Geometry check sheet. Reference: the model listing, model coordinates, mm. Face numbers are marked on the shaded views. Give positions to 0.01 mm unless a question says otherwise; leave off trailing zeros. Write each loop counter-clockwise with the first axis right and the second up, starting at its lowest first coordinate (ties: lowest second). Pieces come first, ordered by that corner, then holes. Notation, with made-up numbers: (65.5, 87) - (106.5, 87) arc R17 cw to (106.5, 118) - close; hole circle Ø10 at (-34.75, -28.75). An arc over 180 degrees is marked (long way). Use a Markdown table: item, result.
```python
from build123d import *

# Parameters (mm, degrees)
BOSS_EXTRUDE1_DEPTH = 5.08
CAVITY2_OUTLINE_R   = 4.59774385
CAVITY2_OUTLINE_R_2 = 13.7414
CAVITY2_DEPTH       = 4.3688
CAVITY2_START       = 3.2512
CAVITY2_2_DEPTH     = 1.1176
CAVITY2_3_OUTLINE_R = 2.794
CAVITY2_3_DEPTH     = 0.7112
SKETCH10_R          = 4.59774385
SKETCH10_R_2        = 2.794
CUT_EXTRUDE1_DEPTH  = 5.08


# Read off the part's stored shape, not the designer's step: Cavity2
with BuildPart() as part:
    # Sketch1 → Boss-Extrude1 (new body)
    with BuildSketch(Plane.XY):
        Polygon((-94.341860078, 47.544254219), (-72.328526744, 47.544254219), (-72.328526744, 52.624254219), (-53.278526744, 52.624254219), (-53.278526744, 47.544254219), (-31.265193411, 47.544254219), (-31.265193411, 52.624254219), (-12.215193411, 52.624254219), (-12.215193411, 47.544254219), (9.798139922, 47.544254219), (9.798139922, 26.589254219), (14.878139922, 26.589254219), (14.878139922, 7.539254219), (9.798139922, 7.539254219), (9.798139922, -13.415745781), (-94.341860078, -13.415745781), (-94.341860078, 7.539254219), (-99.421860078, 7.539254219), (-99.421860078, 26.589254219), (-94.341860078, 26.589254219), align=None)
    extrude(amount=BOSS_EXTRUDE1_DEPTH)

    # Cavity2 outline → Cavity2 (cut)
    with BuildSketch(Plane.XY):
        with Locations((-53.811820296, 33.77125273)):
            Circle(CAVITY2_OUTLINE_R)
        with Locations((-72.649126193, 23.706396)):
            Circle(CAVITY2_OUTLINE_R_2)
    extrude(amount=CAVITY2_DEPTH, mode=Mode.SUBTRACT)

    # Cavity2 2 outline → Cavity2 2 (cut)
    with BuildSketch(Plane.XY.offset(CAVITY2_START)):
        with BuildLine():
            Line((-85.401408895, 28.825513097), (-90.989734661, 27.7567927))
            Line((-90.989734661, 27.7567927), (-88.279765083, 13.586395221))
            Line((-88.279765083, 13.586395221), (-82.945631867, 14.606503426))
            ThreePointArc((-82.945631867, 14.606503426), (-86.190053798, 21.367731092), (-85.401408895, 28.825513097))
        make_face()
    extrude(amount=CAVITY2_2_DEPTH, mode=Mode.SUBTRACT)

    # Cavity2 3 outline → Cavity2 3 (cut)
    with BuildSketch(Plane.XY):
        with Locations((-27.031860078, 2.217954219)):
            Circle(CAVITY2_3_OUTLINE_R)
    extrude(amount=CAVITY2_3_DEPTH, mode=Mode.SUBTRACT)

    # Sketch10 → Cut-Extrude1 (cut)
    with BuildSketch(Plane(origin=(0, 0, 0), x_dir=(-1, 0, 0), z_dir=(0, 0, -1))):
        with Locations((53.811820296, 33.77125273)):
            Circle(SKETCH10_R)
        with Locations((27.031860078, 2.217954219)):
            Circle(SKETCH10_R_2)
        with BuildLine():
            Line((82.945631867, 14.606503426), (88.279765083, 13.586395221))
            Line((88.279765083, 13.586395221), (90.989734661, 27.7567927))
            Line((90.989734661, 27.7567927), (85.401408894, 28.825513097))
            ThreePointArc((85.401408894, 28.825513097), (59.108198587, 26.045060907), (82.945631867, 14.606503426))
        make_face()
    extrude(amount=-CUT_EXTRUDE1_DEPTH, mode=Mode.SUBTRACT)


solid = part.part
```
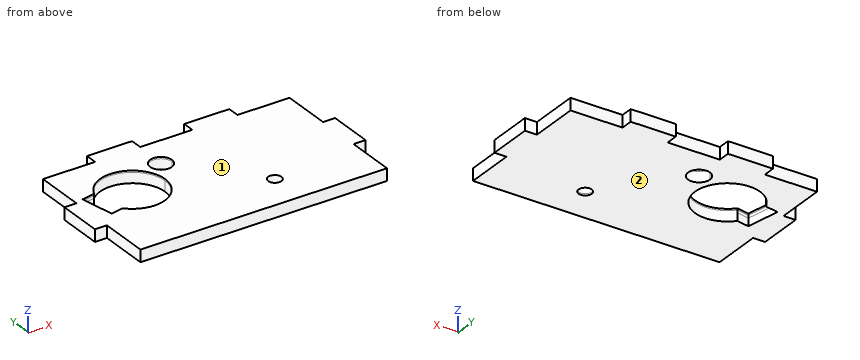
1) Section check D-D on y = 36. Record the boundary of the cut face in (x, z), then the cut area to 3 significant figures.
Working result:
| item | result |
|---|---|
| outline | (-94.34, 0) - (-78.79, 0) - (-78.79, 5.08) - (-94.34, 5.08) - close; (-66.51, 0) - (-57.83, 0) - (-57.83, 5.08) - (-66.51, 5.08) - close; (-49.79, 0) - (9.8, 0) - (9.8, 5.08) - (-49.79, 5.08) - close |
| area | 426 mm² |
2) Mould release check, pull along Z, two halves, no side actions. Record for the marked faces 1 and 2: pulls with the +Z half, pulls with the -Z half, needs draft (parallel to the pull), parting line crosses it, or undercut.
Working result:
| item | result |
|---|---|
| face 1 | pulls with the +Z half |
| face 2 | pulls with the -Z half |
3) Material ranges on L1, parallel to X at y = 49.5, z = 3.65; L2, parallel to X at y = 2, z = 1.35; L3, parallel to X at y = 30, z = 2.1, recorded low to high. Write a range as from..to.
Working result:
| item | result |
|---|---|
| L1 | x = -72.33..-53.28, -31.27..-12.22 |
| L2 | x = -94.34..-29.82, -24.25..9.8 |
| L3 | x = -94.34..-84.86, -60.43..-56.44, -51.18..9.8 |
4) Section check A-A on y = 49. Record the boundary of the cut face in (x, z), then the cut area to 3 significant figures.
Working result:
| item | result |
|---|---|
| outline | (-72.33, 0) - (-53.28, 0) - (-53.28, 5.08) - (-72.33, 5.08) - close; (-31.27, 0) - (-12.22, 0) - (-12.22, 5.08) - (-31.27, 5.08) - close |
| area | 194 mm² |
5) Section check B-B on x = -63. Record the boundary of the cut face in (y, z), then the cut area to 3 significant figures.
Working result:
| item | result |
|---|---|
| outline | (-13.42, 0) - (13.92, 0) - (13.92, 5.08) - (-13.42, 5.08) - close; (33.49, 0) - (52.62, 0) - (52.62, 5.08) - (33.49, 5.08) - close |
| area | 236 mm² |
6) Section check C-C on z = 1.55. Record the boundary of the cut face in (x, y).
Working result:
| item | result |
|---|---|
| outline | (-99.42, 7.54) - (-94.34, 7.54) - (-94.34, -13.42) - (9.8, -13.42) - (9.8, 7.54) - (14.88, 7.54) - (14.88, 26.59) - (9.8, 26.59) - (9.8, 47.54) - (-12.22, 47.54) - (-12.22, 52.62) - (-31.27, 52.62) - (-31.27, 47.54) - (-53.28, 47.54) - (-53.28, 52.62) - (-72.33, 52.62) - (-72.33, 47.54) - (-94.34, 47.54) - (-94.34, 26.59) - (-99.42, 26.59) - close; hole (-90.99, 27.76) - (-88.28, 13.59) - (-82.95, 14.61) arc R13.74 ccw (long way) to (-85.4, 28.83) - close; hole circle Ø9.2 at (-53.81, 33.77); hole circle Ø5.59 at (-27.03, 2.22) |
7) Depth check by flat-ended pin: P1, Ø1.5, axis at x = -97, z = 1.5, coming from the +Y side; P2, Ø2, axis at x = -5.5, z = 3.5, coming from the +Y side; P3, Ø1.5, axis at y = -7.5, z = 2.5, coming from the +X side. Enter the tip coordinate at first touch or a pass-through.
Working result:
| item | result |
|---|---|
| P1 | stops at y = 26.59 |
| P2 | stops at y = 47.54 |
| P3 | stops at x = 9.8 |
